Input: part model. Units: mm. Frame: model coordinates. Face numbers are marked on the shaded views. A direction names the side the tool comes from. Round coordinates to 2 decimals unless told otherwise and drop trailing zeros. Write each loop counter-clockwise with the first axis right and the second up, starting at its lowest first coordinate (ties: lowest second). Pieces come first, ordered by that corner, then holes. Notation, with made-up numbers: (82, 62) - (89, 62) arc R26 cw to (89, 98) - close; hole circle Ø9 at (5.25, 63.25). An arc over 180 degrees is marked (long way). Use one line per item in the form item = value.
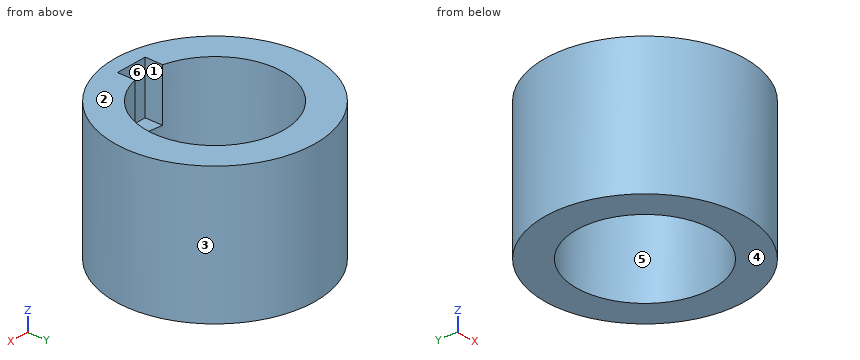
```python
from build123d import *

# Parameters (mm, degrees)
SKETCH1_R               = 9.5
SKETCH1_R_2             = 6.5
BOSS_EXTRUDE1_DEPTH     = 6.5
CUT_EXTRUDE1_REACH      = 24.925
CUT_EXTRUDE1_END_RADIUS = 6.5
CUT_EXTRUDE1_START      = -8
SKETCH2_W               = 3
SKETCH2_H               = 5


with BuildPart() as part:
    # Sketch1 → Boss-Extrude1 (new, symmetric)
    with BuildSketch(Plane.XY):
        with Locations(Location((0, 0, 0), (0, 0, 180))):
            Circle(SKETCH1_R)
        with Locations(Location((0, 0, 0), (0, 0, 180))):
            Circle(SKETCH1_R_2, mode=Mode.SUBTRACT)
    extrude(amount=BOSS_EXTRUDE1_DEPTH, both=True)

    # Cut-Extrude1: up to this cylinder (the profile starts outside it)
    cut_extrude1_end = Plane(origin=(0, 0, 4), z_dir=(0, 0, -1)) * Cylinder(CUT_EXTRUDE1_END_RADIUS, 63.85, mode=Mode.PRIVATE)
    # Sketch2 → Cut-Extrude1 (cut, up to the surface)
    with BuildSketch(Plane(origin=(0, 0, 0), x_dir=(1, 0, 0), z_dir=(0, 1, 0)).offset(CUT_EXTRUDE1_START), mode=Mode.PRIVATE) as cut_extrude1_sk1:
        with Locations((0, -4)):
            Rectangle(SKETCH2_W, SKETCH2_H)
    cut_extrude1_tool1 = extrude(cut_extrude1_sk1.sketch, amount=CUT_EXTRUDE1_REACH, mode=Mode.PRIVATE) - cut_extrude1_end
    add(cut_extrude1_tool1.solids().sort_by_distance((0, -8, 4))[0], mode=Mode.SUBTRACT)


solid = part.part
```
(1) Cut plane A-A on x = 0. Output: boundary loops of the cut face in (y, z).
Derived:
outline = (-9.5, -6.5) - (-6.5, -6.5) - (-6.5, 1.5) - (-8, 1.5) - (-8, 6.5) - (-9.5, 6.5) - close; (6.5, -6.5) - (9.5, -6.5) - (9.5, 6.5) - (6.5, 6.5) - close
(2) Material intervals for L1, parallel to Y at x = 0, z = 3.5; L2, parallel to Y at x = 0, z = -0.75; L3, parallel to X at y = 2.5, z = 2.25, sorted ascending.
Derived:
L1 = -9.5 to -8, 6.5 to 9.5
L2 = -9.5 to -6.5, 6.5 to 9.5
L3 = -9.17 to -6, 6 to 9.17
(3) Cut plane C-C on z = 2.25. Output: boundary loops of the cut face in (x, y).
Derived:
outline = circle Ø19 at (0, 0); hole (-1.5, -8) - (1.5, -8) - (1.5, -6.32) arc R6.5 ccw (long way) to (-1.5, -6.32) - close
(4) Draft query along X for the marked faces 3, 4, 5 and 6. Return one class per face: released by +X, released by -X, zero draft, split by the parting line, or undercut.
Derived:
face_3 = split by the parting line
face_4 = zero draft
face_5 = undercut
face_6 = undercut
(5) First-contact query: pin 1 Ø4 at (y, z) = (-5.5, -2) entering from -X; pin 2 Ø0.5 at (y, z) = (-7, 3) entering from +X; pin 3 Ø5 at (x, z) = (6.5, 2) entering from +Y. Flat tips, straight axial feed; report the tip coordinate or a pass-through.
Derived:
pin_1 = -8.83
pin_2 = 6.68
pin_3 = 8.62
(6) Access query for the marked faces 1 and 2. Directions: +Z, -Z, +X, -X, +Y, -Y. A direction counts if a zero-diameter tool reaches every point of the face in a straight line with its end or side. Return the directions, or none.
Derived:
face_1 = +Z
face_2 = +Z, +X, -X, +Y, -Y
(7) Cut plane D-D on y = -4. Output: boundary loops of the cut face in (x, z).
Derived:
outline = (-8.62, -6.5) - (-5.12, -6.5) - (-5.12, 6.5) - (-8.62, 6.5) - close; (5.12, -6.5) - (8.62, -6.5) - (8.62, 6.5) - (5.12, 6.5) - close
(8) Cut plane B-B on y = 0. Output: boundary loops of the cut face in (x, z).
Derived:
outline = (-9.5, -6.5) - (-6.5, -6.5) - (-6.5, 6.5) - (-9.5, 6.5) - close; (6.5, -6.5) - (9.5, -6.5) - (9.5, 6.5) - (6.5, 6.5) - close
